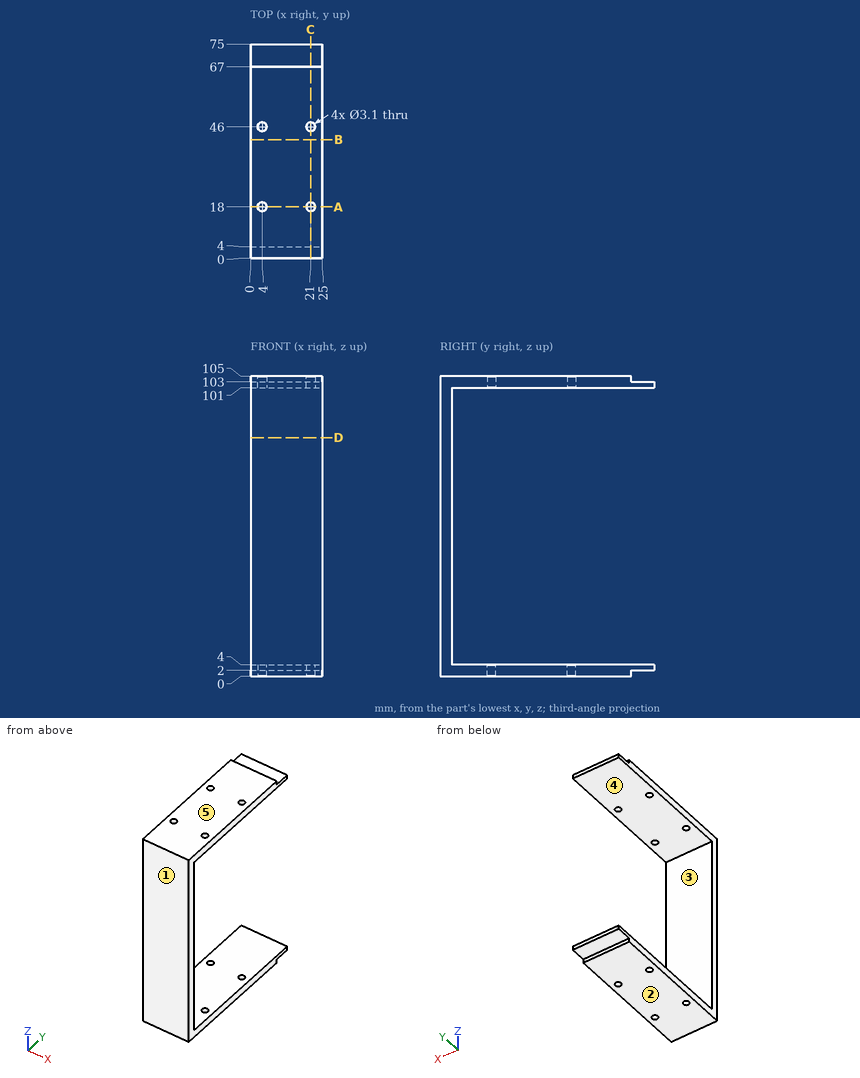
Answer from the drawing. Dimensions are ordinates in mm from the lowest x, y and z of the part. A direction names the side the tool comes from. Round coordinates to 2 decimals unless told otherwise and drop trailing zeros. Loops run counter-clockwise (first coordinate to the right, second up) from the corner with the lowest first, then second, coordinate; pieces in that order, holes last.
1) A cutting plane is placed at C-C on x = 21. Determine the outline of the cut face in (y, z), plus the area to 3 significant figures.
Outcome:
outline: (0, 0) - (16.45, 0) - (16.45, 4) - (4, 4) - (4, 101) - (16.45, 101) - (16.45, 105) - (0, 105) - close; (19.55, 0) - (44.45, 0) - (44.45, 4) - (19.55, 4) - close; (19.55, 101) - (44.45, 101) - (44.45, 105) - (19.55, 105) - close; (47.55, 0) - (67, 0) - (67, 2) - (75, 2) - (75, 4) - (47.55, 4) - close; (47.55, 101) - (75, 101) - (75, 103) - (67, 103) - (67, 105) - (47.55, 105) - close
area: 906 mm2
2) A cutting plane is placed at A-A on y = 18. Determine the outline of the cut face in (x, z).
Outcome:
outline: (0, 0) - (2.45, 0) - (2.45, 4) - (0, 4) - close; (0, 101) - (2.45, 101) - (2.45, 105) - (0, 105) - close; (5.55, 0) - (19.45, 0) - (19.45, 4) - (5.55, 4) - close; (5.55, 101) - (19.45, 101) - (19.45, 105) - (5.55, 105) - close; (22.55, 0) - (25, 0) - (25, 4) - (22.55, 4) - close; (22.55, 101) - (25, 101) - (25, 105) - (22.55, 105) - close
3) A cutting plane is placed at D-D on z = 83.5. Determine the outline of the cut face in (x, y), plus the area to 3 significant figures.
Outcome:
outline: (0, 0) - (25, 0) - (25, 4) - (0, 4) - close
area: 100 mm2
4) For a pull along Z with two mould halves and no side action, classify the marked faces 1, 2 and 3 as released by +Z, released by -Z, zero draft, split by the parting line, or undercut.
Outcome:
face 1: zero draft
face 2: released by -Z
face 3: undercut
5) For the marked faces 4 and 5, determine the directions among +Z, -Z, +X, -X, +Y, -Y from which every point of the face is accessible in a straight line to the end or side of a thin tool.
Outcome:
face 4: +X, -X, +Y
face 5: +Z, +X, -X, +Y, -Y
6) Consider line 1 (Y direction, x = 21, z = 1); line 2 (Y direction, x = 21, z = 3.25); line 3 (X direction, y = 18, z = 2.1). Determine where each line is inside the solid, lowest interval first.
Outcome:
line 1: y = 0 to 16.45, 19.55 to 44.45, 47.55 to 67
line 2: y = 0 to 16.45, 19.55 to 44.45, 47.55 to 75
line 3: x = 0 to 2.45, 5.55 to 19.45, 22.55 to 25
7) Given P1, Ø1, axis at x = 12.5, z = 104.5, coming from the +Y side; P2, Ø12, axis at x = 21.5, z = 38, coming from the +Y side; P3, Ø2.5, axis at x = 13.5, y = 69.5, coming from the -Z side, each flat-ended and moving along its own axis, determine where each tip first touches the part or whether it passes through.
Outcome:
P1: stops at y = 67
P2: stops at y = 4
P3: stops at z = 2
8) A cutting plane is placed at B-B on y = 41.5. Determine the outline of the cut face in (x, z), plus the area to 3 significant figures.
Outcome:
outline: (0, 0) - (25, 0) - (25, 4) - (0, 4) - close; (0, 101) - (25, 101) - (25, 105) - (0, 105) - close
area: 200 mm2
